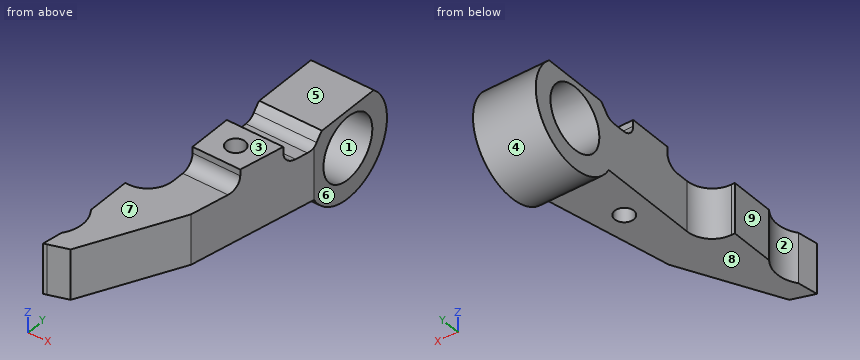
from build123d import *

# Parameters (mm, degrees)
BOSS_EXTRU_1_DEPTH           = 8
CONG_1_R                     = 4
ESQUISSE2_R                  = 5
ENL_V_MAT_EXTRU_1_DEPTH      = 9
BOSS_EXTRU_2_DEPTH           = 8
ESQUISSE4_R                  = 5
BOSS_EXTRU_3_DEPTH           = 10
ENL_V_MAT_EXTRU_2_DEPTH      = 1
ENL_V_MAT_EXTRU_2_DEPTH_BACK = 16
BOSS_EXTRU_4_DEPTH           = 3
CONG_2_R                     = 2
ESQUISSE7_R                  = 1.5
ENL_V_MAT_EXTRU_3_DEPTH      = 16


with BuildPart() as part:
    # Esquisse1 → Boss.-Extru.1 (new body)
    with BuildSketch(Plane.XY):
        Polygon((0, 0), (10, 0), (6, -20), (-1.5, -35), (-4.5, -36), (-4.5, -20), (0, -20), align=None)
    extrude(amount=BOSS_EXTRU_1_DEPTH)

    # Congé1
    cong_1_edges = [part.edges().sort_by_distance(p)[0] for p in [
        (0, -20, 4),
    ]]
    fillet(cong_1_edges, radius=CONG_1_R)

    # Esquisse2 → Enlèv. mat.-Extru.1 (cut, through all)
    with BuildSketch(Plane.XY.offset(8)):
        with Locations((-8.5, -30)):
            Circle(ESQUISSE2_R)
    extrude(amount=-ENL_V_MAT_EXTRU_1_DEPTH, mode=Mode.SUBTRACT)

    # Esquisse3 → Boss.-Extru.2 (add)
    with BuildSketch(Plane.XY.offset(8)):
        Polygon((-4.5, -33), (-5, -36.166666667), (-4.5, -36), align=None)
    extrude(amount=-BOSS_EXTRU_2_DEPTH)

    # Esquisse4 → Boss.-Extru.3 (add)
    with BuildSketch(Plane.ZY):
        with BuildLine():
            Line((8, 0), (0, 0))
            ThreePointArc((0, 0), (4, 14.92820323), (8, 0))
        make_face()
        with Locations((4, 6.92820323)):
            Circle(ESQUISSE4_R, mode=Mode.SUBTRACT)
    extrude(amount=-BOSS_EXTRU_3_DEPTH)

    # Esquisse5 → Enlèv. mat.-Extru.2 (cut, two sides)
    with BuildSketch(Plane(origin=(10, 0, 0), x_dir=(0, 0, -1), z_dir=(1, 0, 0))) as enl_v_mat_extru_2_sk:
        Polygon((-10, 122.961773442), (-10, 12.219705852), (-10, 1.636700608), (-10, -109.105366981), (-231.484135179, -109.105366981), (-231.484135179, 122.961773442), align=None)
    extrude(amount=ENL_V_MAT_EXTRU_2_DEPTH, mode=Mode.SUBTRACT)
    extrude(enl_v_mat_extru_2_sk.sketch, amount=-ENL_V_MAT_EXTRU_2_DEPTH_BACK, mode=Mode.SUBTRACT)

    # Esquisse6 → Boss.-Extru.4 (add)
    with BuildSketch(Plane.XY.offset(8)):
        Polygon((0, -5), (0, -12), (7.6, -12), (9, -5), align=None)
    extrude(amount=BOSS_EXTRU_4_DEPTH)

    # Congé2
    cong_2_edges = [part.edges().sort_by_distance(p)[0] for p in [
        (5, 0, 8),
        (4.5, -5, 8),
        (3.8, -12, 8),
    ]]
    fillet(cong_2_edges, radius=CONG_2_R)

    # Esquisse7 → Enlèv. mat.-Extru.3 (cut, through all)
    with BuildSketch(Plane.XY.offset(11)):
        with Locations((4.15, -8.5)):
            Circle(ESQUISSE7_R)
    extrude(amount=-ENL_V_MAT_EXTRU_3_DEPTH, mode=Mode.SUBTRACT)


solid = part.part
Can you work these out from the model? Positions are in its coordinate system, mm. Face numbers are marked on the shaded views. A direction names the side the tool comes from. Give positions to 0.01 mm unless a question says otherwise; leave off trailing zeros. Loops run counter-clockwise (first coordinate to the right, second up) from the corner with the lowest first, then second, coordinate; pieces in that order, holes last. Notation, with made-up numbers: (-28.5, -25) -> (11.5, -25) arc R18 cw to (11.5, -7) -> close; hole circle Ø2 at (89, 27). An arc over 180 degrees is marked (long way). Return JSON: item names as keys, results as strings.
Q1. On a 3-axis mill with a long thin cutter (end or side, diameter ignored), from which of +Z, -Z, +X, -X, +Y, -Y can I reach the whole of each face in a straight line? I mean the marked faces 5, 6, 7, 8 and 9. Say none if no direction works.
Checks:
{"face 5": "+Z, +X, -X, +Y", "face 6": "+Z, -Z, +X, +Y, -Y", "face 7": "+Z, +X, -X, -Y", "face 8": "-Z, +X, -X, -Y", "face 9": "+Z, -Z, -X, +Y"}
Q2. For pin 1 Ø1.1 at (x, z) = (5.5, 10.5) entering from -Y; pin 2 Ø2 at (x, y) = (7.5, 0) entering from -Z; pin 3 Ø1.5 at (x, z) = (4, -2) entering from +Y, each with a flat end and sliding along its axis, tell me the tip position at first contact or that it passes through.
Checks:
{"pin 1": "stops at y = -12", "pin 2": "stops at z = -1.37", "pin 3": "stops at y = 12.96"}
Q3. I want a section at A-A, the plane z = 4. List the corners of the cut face in (x, y) for me.
Checks:
{"outline": "(-5, -36.17) -> (-1.5, -35) -> (6, -20) -> (10, 0) -> (10, 1.93) -> (0, 1.93) -> (0, -16) arc R4 cw to (-4, -20) -> (-4.5, -20) -> (-4.5, -27) arc R5 cw to (-4.5, -33) -> close; (0, 11.93) -> (10, 11.93) -> (10, 14.93) -> (0, 14.93) -> close; hole circle Ø3 at (4.15, -8.5)"}
Q4. We'd pull the mould along Y, two halves only. Please class the marked faces 1, 2, 3 and 4: released by +Y, released by -Y, zero draft, split by the parting line, or undercut.
Checks:
{"face 1": "undercut", "face 2": "undercut", "face 3": "zero draft", "face 4": "split by the parting line"}
Q5. I need wall thicknesses on probe 1 along Y at (x, z) = (4.15, 3.5); probe 2 along Y at (x, z) = (4.5, 4); probe 3 along X at (y, z) = (9.5, 9.5). Which ranges of each line are inside material? Lowest first, please.
Checks:
{"probe 1": "y = -23.7 to -10, -7 to 1.95, 11.9 to 14.91", "probe 2": "y = -23 to -9.96, -7.04 to 1.93, 11.93 to 14.93", "probe 3": "x = 0 to 10"}
Q6. I want a section at C-C, the plane x = 4. List the corners of the cut face in (y, z) for me, then the cut area to 3 significant figures.
Checks:
{"outline": "(-24, 0) -> (-9.99, 0) -> (-9.99, 11) -> (-12, 11) -> (-12, 10) arc R2 cw to (-14, 8) -> (-24, 8) -> close; (-7.01, 0) -> (0, 0) arc R8 ccw (long way) to (12.22, 10) -> (1.64, 10) arc R8 ccw to (0.53, 8.8) arc R2 cw to (-1.07, 8) -> (-3, 8) arc R2 cw to (-5, 10) -> (-5, 11) -> (-7.01, 11) -> close; hole circle Ø10 at (6.93, 4)", "area": "284 mm2"}
Q7. I want a section at B-B, the plane y = -8.5. List the corners of the cut face in (x, z) for me, then the cut area to 3 significant figures.
Checks:
{"outline": "(0, 0) -> (2.65, 0) -> (2.65, 11) -> (0, 11) -> close; (5.65, 0) -> (8.3, 0) -> (8.3, 11) -> (5.65, 11) -> close", "area": "58.3 mm2"}
Q8. I want a section at D-D, the plane x = 0.5. List the corners of the cut face in (y, z) for me.
Checks:
{"outline": "(-31, 0) -> (0, 0) arc R8 ccw (long way) to (12.22, 10) -> (1.64, 10) arc R8 ccw to (0.53, 8.8) arc R2 cw to (-1.07, 8) -> (-3, 8) arc R2 cw to (-5, 10) -> (-5, 11) -> (-12, 11) -> (-12, 10) arc R2 cw to (-14, 8) -> (-31, 8) -> close; hole circle Ø10 at (6.93, 4)"}
